from build123d import *

# Parameters (mm, degrees)
SKETCH1_W            = 29.9
SKETCH1_H            = 10.3
SKETCH1_R            = 2.4
BOSS_EXTRUDE1_DEPTH  = 30
BOSS_EXTRUDE3_START  = -2
SKETCH4_W            = 29.9
SKETCH4_H            = 10.3
BOSS_EXTRUDE3_DEPTH  = 28
SKETCH2_W            = 18.9
SKETCH2_H            = 23
CUT_EXTRUDE1_DEPTH   = 38.631801711
SKETCH3_W            = 0.65
SKETCH3_H            = 3
CUT_EXTRUDE2_DEPTH   = 37.559335333
M3_CLEARANCE_HOLE1_D = 3.6
FILLET1_R            = 1.5
CHAMFER1_SIZE        = 0.6


with BuildPart() as part:
    # Sketch1 → Boss-Extrude1 (new body)
    with BuildSketch(Plane(origin=(0, 0, 0), x_dir=(1, 0, 0), z_dir=(0, 1, 0))):
        with Locations((-5.3, 0)):
            Rectangle(SKETCH1_W, SKETCH1_H)
        with Locations(Location((0, 0, 0), (0, 0, 270))):
            Circle(SKETCH1_R, mode=Mode.SUBTRACT)
        with Locations(Location((-14.25, 0, 0), (0, 0, 270))):
            Circle(SKETCH1_R, mode=Mode.SUBTRACT)
    extrude(amount=BOSS_EXTRUDE1_DEPTH)

    # Sketch4 → Boss-Extrude3 (add)
    with BuildSketch(Plane.XZ.offset(BOSS_EXTRUDE3_START)):
        with Locations((-5.3, 0)):
            Rectangle(SKETCH4_W, SKETCH4_H)
    extrude(amount=-BOSS_EXTRUDE3_DEPTH)

    # Sketch2 → Cut-Extrude1 (cut, through all)
    with BuildSketch(Plane.XY.offset(5.15)):
        with Locations((-10.8, 18.5)):
            Rectangle(SKETCH2_W, SKETCH2_H)
    extrude(amount=-CUT_EXTRUDE1_DEPTH, mode=Mode.SUBTRACT)

    # Sketch3 → Cut-Extrude2 (cut, through all)
    with BuildSketch(Plane.XZ):
        with Locations((-11.625, 0)):
            Rectangle(SKETCH3_W, SKETCH3_H)
        with Locations((-2.625, 0)):
            Rectangle(SKETCH3_W, SKETCH3_H)
    extrude(amount=-CUT_EXTRUDE2_DEPTH, mode=Mode.SUBTRACT)

    # M3 Clearance Hole1 (through all)
    with Locations(Plane.XY.offset(5.15)):
        with Locations((4.65, 12), (4.65, 27)):
            Hole(M3_CLEARANCE_HOLE1_D / 2)

    # Fillet1
    # the kernel refuses this fillet: 1.5 mm, written as the material it takes off along each edge
    with BuildSketch(Plane(origin=(-2.3, 2, 0.68556546), x_dir=(0.5486256089659476, 0, 0.8360681438655243), z_dir=(0, -1, 0)), Plane(origin=(-11.95, 2, -0.68556546), x_dir=(-0.5486256089659476, 0, -0.8360681438655244), z_dir=(0, -1, 0))) as fillet1_piece_1:
        with BuildLine():
            CenterArc((1.80773108, 1.436922187), FILLET1_R, 221.305086591, 32.01998054)
            Line((0.680922774, 0.446819645), (0, 0))
            ThreePointArc((0, 0), (0.688659459, 0.100924501), (1.377318918, 0))
        make_face()
    extrude(amount=5.443297295, mode=Mode.SUBTRACT)
    with BuildSketch(Plane(origin=(-2.3, 2, -0.68556546), x_dir=(0.5486256089659476, 0, -0.8360681438655245), z_dir=(0, -1, 0)), Plane(origin=(-11.95, 2, 0.68556546), x_dir=(-0.5486256089659488, 0, 0.8360681438655235), z_dir=(0, -1, 0))) as fillet1_piece_2:
        with BuildLine():
            CenterArc((1.80773108, -1.436922187), FILLET1_R, 106.67493287, 32.01998054)
            Line((0.680922774, -0.446819645), (0, 0))
            ThreePointArc((0, 0), (0.688659459, -0.100924501), (1.377318918, 0))
        make_face()
    extrude(amount=5.443297295, mode=Mode.SUBTRACT)

    # Chamfer1
    chamfer1_edges = [part.edges().sort_by_distance(p)[0] for p in [
        (2.4, 0, 0),
        (-16.65, 0, 0),
        (-12.351519212, 0, 1.61541677),
        (-12.351519212, 0, -1.61541677),
        (-1.898480788, 0, 1.61541677),
        (-1.898480788, 0, -1.61541677),
        (-5.3, 0, -5.15),
        (9.65, 0, 0),
        (-5.3, 0, 5.15),
        (-20.25, 0, 0),
        (-11.625, 0, -1.5),
        (-11.3, 0, 0),
        (-11.625, 0, 1.5),
        (-2.625, 0, 1.5),
        (-2.95, 0, 0),
        (-2.625, 0, -1.5),
    ]]
    chamfer(chamfer1_edges, length=CHAMFER1_SIZE)


solid = part.part
Build history of the part. All positions in model axes, mm. A direction names the side the tool comes from. Coordinates: 2 decimals unless noted, no trailing zeros. Write each loop counter-clockwise with the first axis right and the second up, starting at its lowest first coordinate (ties: lowest second). Pieces come first, ordered by that corner, then holes.
(1) Cut at B-B on z = 3.75. List the corners of the cut face in (x, y).
(2) Cut at D-D on x = 0. List the corners of the cut face in (y, z), and give its area (3 significant figures).
(3) Mould opens along Z. For faces 1 (the flat face through (0, 2, 0)), 2 (the flat face through (-6, 0, 0)), 3 (the flat face through (1, 12, -5.15)) say: pulls with the +Z half, pulls with the -Z half, needs draft (parallel to the pull), parting line crosses it, or undercut.
(4) 3-axis set-ups, long thin cutter, end or side, ignore diameter. For faces 4 (the flat face through (-2.95, 4, 0)), 5 (the flat face through (-14, 2, 0)), 6 (the flat face through (-1.35, 18, 0)), 7 (the flat face through (-20.25, 4, 0)), 8 (the flat face through (1, 12, 5.15)): which of +Z, -Z, +X, -X, +Y, -Y reach the whole face in a straight line?
(5) Pin check, flat tips, straight feed: pin 1 Ø12 at (x, y) = (-4.5, 12) entering from +Z; pin 2 Ø3 at (x, z) = (-11, 2.5) entering from +Y; pin 3 Ø5 at (y, z) = (25, 0) entering from -X; pin 4 Ø1.4 at (x, z) = (-0.5, -1) entering from -Y. Stop position of each tip, or through.
(6) Cut at C-C on y = 27. List the corners of the cut face in (x, z).
(7) Drill centre lines: line 1 (Y direction, x = 4.65, z = -2.5); line 2 (Y direction, x = 3.25, z = 1.5); line 3 (Z direction, x = -14.25, y = 1.1). Where is each one in solid material? Low to high.
(8) Cut at A-A on x = 4.65. List the corners of the cut face in (y, z).
Working result:
1. outline: (-20.25, 0.6) - (-19.65, 0) - (9.05, 0) - (9.65, 0.6) - (9.65, 30) - (-1.35, 30) - (-1.35, 7) - (-20.25, 7) - close; hole circle Ø3.6 at (4.65, 12); hole circle Ø3.6 at (4.65, 27)
2. outline: (0, -4.55) - (0.6, -5.15) - (30, -5.15) - (30, 5.15) - (0.6, 5.15) - (0, 4.55) - (0, 3) - (0.6, 2.4) - (2, 2.4) - (2, -2.4) - (0.6, -2.4) - (0, -3) - close
2. area: 299 mm2
3. face 1: undercut
3. face 2: needs draft
3. face 3: pulls with the -Z half
4. face 4: +Y, -Y
4. face 5: -Y
4. face 6: +Z, -Z, -X, +Y
4. face 7: +Z, -Z, -X, +Y, -Y
4. face 8: +Z, +X, -X, +Y, -Y
5. pin 1: stops at z = 5.15
5. pin 2: stops at y = 7
5. pin 3: stops at x = -1.35
5. pin 4: stops at y = 2
6. outline: (-1.35, -5.15) - (2.85, -5.15) - (2.85, 5.15) - (-1.35, 5.15) - close; (6.45, -5.15) - (9.65, -5.15) - (9.65, 5.15) - (6.45, 5.15) - close
7. line 1: y = 0 to 10.2, 13.8 to 25.2, 28.8 to 30
7. line 2: y = 0 to 10.87, 13.13 to 25.87, 28.13 to 30
7. line 3: z = -5.15 to -2.4, 2.4 to 5.15
8. outline: (0, -4.55) - (0.6, -5.15) - (10.2, -5.15) - (10.2, 5.15) - (0.6, 5.15) - (0, 4.55) - close; (13.8, -5.15) - (25.2, -5.15) - (25.2, 5.15) - (13.8, 5.15) - close; (28.8, -5.15) - (30, -5.15) - (30, 5.15) - (28.8, 5.15) - close
